from build123d import *

# Parameters (mm, degrees)
ESQUISSE2_W             = 2
ESQUISSE2_H             = 44.5
ENL_V_MAT_EXTRU_1_DEPTH = 32.25


with BuildPart() as part:
    # Esquisse1 → Révolution1 (revolve)
    with BuildSketch(Plane(origin=(0, 0, 0), x_dir=(0, 0, -1), z_dir=(1, 0, 0))):
        Polygon((25, 44.5), (25, 0), (31.25, 0), (31.25, 4.5), (28, 4.5), (28, 44.5), align=None)
    revolve(axis=Axis((0, 0, 0), (0, 1, 0)))

    # Esquisse2 → Enlèv. mat.-Extru.1 (cut, through all)
    with BuildSketch(Plane.XY):
        with Locations((0, 22.25)):
            Rectangle(ESQUISSE2_W, ESQUISSE2_H)
    extrude(amount=-ENL_V_MAT_EXTRU_1_DEPTH, mode=Mode.SUBTRACT)


solid = part.part
The model under review builds one solid part; all positions refer to its coordinate system, in mm. A direction names the side the tool comes from. Coordinates: 2 decimals unless noted, no trailing zeros. Loops run counter-clockwise (first coordinate to the right, second up) from the corner with the lowest first, then second, coordinate; pieces in that order, holes last.
(1) Wall thickness on L1, parallel to X at y = 24, z = 0; L2, parallel to Y at x = 23, z = -17; L3, parallel to X at y = 24, z = -21: over which ranges is each line inside the solid? List them lowest first.
Determined:
L1: x = -28 to -25, 25 to 28
L2: y = 0 to 4.5
L3: x = -18.52 to -13.56, 13.56 to 18.52
(2) Consider section C-C, the plane x = 0. Give the boundary of the cut face in (y, z).
Determined:
outline: (0, 25) - (44.5, 25) - (44.5, 28) - (4.5, 28) - (4.5, 31.25) - (0, 31.25) - close
(3) Consider section B-B, the plane z = 0. Give the boundary of the cut face in (x, y), plus the area to 3 significant figures.
Determined:
outline: (-31.25, 0) - (-25, 0) - (-25, 44.5) - (-28, 44.5) - (-28, 4.5) - (-31.25, 4.5) - close; (25, 0) - (31.25, 0) - (31.25, 4.5) - (28, 4.5) - (28, 44.5) - (25, 44.5) - close
area: 296 mm2
(4) Insertion check: P1, Ø10, axis at y = 13, z = -1.5, coming from the +X side; P2, Ø3, axis at y = 24.5, z = 3, coming from the -X side; P3, Ø12, axis at y = 11, z = 9.5, coming from the -X side. Each pin has a flat end and moves straight along its axis. Give the tip position at first contact, or say it passes through.
Determined:
P1: stops at x = 28
P2: stops at x = -27.96
P3: stops at x = -27.78
(5) Tool access review of faces 1 (the cylindrical face through (-1.36, 2.28, 31.22)), 2 (the cylindrical face through (-1.217, 24.78, 27.974)), 3 (the flat face through (-1, 22, -27)): name each direction out of +Z, -Z, +X, -X, +Y, -Y from which nothing blocks a thin tool from reaching the whole face with its end or side.
Determined:
face 1: +Y, -Y
face 2: +Y
face 3: -Z, +Y, -Y
(6) Consider section D-D, the plane y = 11. Give the boundary of the cut face in (x, z), plus the area to 3 significant figures.
Determined:
outline: (-1, -27.98) - (-1, -24.98) arc R25 cw (long way) to (1, -24.98) - (1, -27.98) arc R28 ccw (long way) to start
area: 494 mm2
(7) Consider section A-A, the plane x = 22. Give the boundary of the cut face in (y, z).
Determined:
outline: (0, -22.19) - (4.5, -22.19) - (4.5, -17.32) - (44.5, -17.32) - (44.5, -11.87) - (0, -11.87) - close; (0, 11.87) - (44.5, 11.87) - (44.5, 17.32) - (4.5, 17.32) - (4.5, 22.19) - (0, 22.19) - close
